Could you check a few things on this model? Use its own coordinates, in mm. A direction names the side the tool comes from. Round coordinates to 2 decimals unless told otherwise and drop trailing zeros. Loops run counter-clockwise (first coordinate to the right, second up) from the corner with the lowest first, then second, coordinate; pieces in that order, holes last. Notation, with made-up numbers: (78, -38) -> (106, -38) arc R12 cw to (106, -19) -> close; hole circle Ø11 at (35, 0). An arc over 180 degrees is marked (long way). One line per item, written item: value.
```python
from build123d import *

# Parameters (mm, degrees)
F0_R        = 20
F0_R_2      = 7.5
F1_DEPTH    = 150
F2_W        = 25
F2_H        = 25
F3_DEPTH    = 100
F4_T        = 2.5
F4_T3_DEPTH = 105
F4_T5_DEPTH = 30
F4_T7_DEPTH = 30


# Not quite as in the source:
# - a shell that OpenCascade refuses in one call is made with other operations: the cavity is built on its own and cut out
# - a feature names something its author has since deleted; it is built from what else it names


with BuildPart() as f1:
    # F0 (on Top) → F1 (new body)
    with BuildSketch(Plane.XY):
        Circle(F0_R)
        Circle(F0_R_2, mode=Mode.SUBTRACT)
        Circle(F0_R_2)
    extrude(amount=F1_DEPTH)

    # F2 (on face) → F3 (cut)
    with BuildSketch(Plane.XY.offset(150)):
        Rectangle(F2_W, F2_H)
    extrude(amount=-F3_DEPTH, mode=Mode.SUBTRACT)

    # F4: shell of thickness 2.5, made by hand


with BuildPart() as f4_core1:
    # F4_t2: copy of F1
    add(f1.part)

    # the walls: a layer under each face that stays
    f4_faces = [f4_core1.faces().sort_by_distance(p)[0] for p in [
        (-20, 0, 75),
        (-13.3333333333, -13.3333333333, 150),
        (-12.5, 0, 100),
        (0, -12.5, 100),
        (12.5, 0, 100),
        (0, 12.5, 100),
        (0, 0, 50),
    ]]
    thicken(f4_faces, amount=-F4_T, mode=Mode.SUBTRACT)

    # F4_s4 → F4_t3 (cut)
    with BuildSketch(Plane.XY.offset(47.5)):
        Polygon((-12.475, 12.475), (-15, 12.5), (-15, 15), (-12.5, 15), align=None)
        Polygon((-12.475, -12.475), (-15, -12.5), (-15, -15), (-12.5, -15), align=None)
        Polygon((12.475, -12.475), (12.5, -15), (15, -15), (15, -12.5), align=None)
        Polygon((12.475, 12.475), (15, 12.5), (15, 15), (12.5, 15), align=None)
    extrude(amount=F4_T3_DEPTH, mode=Mode.SUBTRACT)

    # F4_s6 → F4_t5 (cut)
    with BuildSketch(Plane.XZ.offset(-15)):
        Polygon((-12.475, 50.025), (-15, 50), (-15, 47.5), (-12.5, 47.5), align=None)
        Polygon((12.475, 50.025), (15, 50), (15, 47.5), (12.5, 47.5), align=None)
    extrude(amount=F4_T5_DEPTH, mode=Mode.SUBTRACT)

    # F4_s8 → F4_t7 (cut)
    with BuildSketch(Plane.YZ.offset(-15)):
        Polygon((-12.475, 50.025), (-15, 50), (-15, 47.5), (-12.5, 47.5), align=None)
        Polygon((12.475, 50.025), (15, 50), (15, 47.5), (12.5, 47.5), align=None)
    extrude(amount=F4_T7_DEPTH, mode=Mode.SUBTRACT)


with BuildPart() as f1_1:
    add(f1.part)

    # what is left inside the walls is the cavity
    f4_cavity = [f4_core1.part.solids().sort_by_distance(p)[0] for p in [
        (-17.475, 0, 98.333333),
    ]]
    add(f4_cavity, mode=Mode.SUBTRACT)


solid = f1_1.part
```
(1) For pin 1 Ø2 at (x, y) = (-1.5, 13.5) entering from -Z; pin 2 Ø12 at (x, y) = (5.5, -2) entering from +Z; pin 3 Ø20 at (x, z) = (2.5, 92.5) entering from +Y, each with a flat end and sliding along its axis, tell me the tip position at first contact or that it passes through.
Results below:
pin 1: stops at z = 47.5
pin 2: stops at z = 50
pin 3: stops at y = 20
(2) We'd pull the mould along Y, two halves only. Please class faces 1 (the face through (-4.336, -19.524, 73.95)), 2 (the face through (16, 0, 147.5)), 3 (the face through (0, -18, 0)): +Y half, -Y half, draft (parallel to the pull), parting line (faces both ways), or undercut.
Results below:
face 1: parting line
face 2: undercut
face 3: draft
(3) Imagine slicing it at A-A on z = 73.5. Write out the boundary of the cut face in (x, y), then the cut area to 3 significant figures.
Results below:
outline: circle Ø40 at (0, 0); hole (-15, -9.01) -> (-15, 9.01) arc R17.5 ccw to start; hole (-12.5, -12.5) -> (12.5, -12.5) -> (12.5, 12.5) -> (-12.5, 12.5) -> close; hole (-9.01, -15) arc R17.5 ccw to (9.01, -15) -> close; hole (-9.01, 15) -> (9.01, 15) arc R17.5 ccw to start; hole (15, -9.01) arc R17.5 ccw to (15, 9.01) -> close
area: 510 mm²
(4) Please list where these lines run through material, in increasing order: L1, parallel to Y at x = 0, z = 68; L2, parallel to Y at x = 0, z = 43.5; L3, parallel to X at y = -3, z = 63.
Results below:
L1: y = -20 to -17.5, -15 to -12.5, 12.5 to 15, 17.5 to 20
L2: y = -20 to -17.5, 17.5 to 20
L3: x = -19.77 to -17.24, -15 to -12.5, 12.5 to 15, 17.24 to 19.77
(5) On a 3-axis mill with a long thin cutter (end or side, diameter ignored), from which of +Z, -Z, +X, -X, +Y, -Y can I reach the whole of each face in a straight line? I mean faces 4 (the face through (0, -15, 98)), 5 (the face through (0, -12.5, 101)), 6 (the face through (13, 0, 150)). Say none if no direction works.
Results below:
face 4: -Z
face 5: +Z
face 6: +Z, +X, -X, +Y, -Y
(6) Imagine slicing it at D-D on z = 36.5. Write out the boundary of the cut face in (x, y), then the cut area to 3 significant figures.
Results below:
outline: circle Ø40 at (0, 0); hole circle Ø35 at (0, 0)
area: 295 mm²
(7) Imagine slicing it at B-B on x = 0. Write out the boundary of the cut face in (y, z), then the cut area to 3 significant figures.
Results below:
outline: (-20, 0) -> (-17.5, 0) -> (-17.5, 147.5) -> (-15, 147.5) -> (-15, 47.5) -> (15, 47.5) -> (15, 147.5) -> (17.5, 147.5) -> (17.5, 0) -> (20, 0) -> (20, 150) -> (12.5, 150) -> (12.5, 50) -> (-12.5, 50) -> (-12.5, 150) -> (-20, 150) -> close
area: 1,340 mm²
